Can you work these out from the model? Positions are in its coordinate system, mm. A direction names the side the tool comes from. Give positions to 0.01 mm unless a question says otherwise; leave off trailing zeros. Loops run counter-clockwise (first coordinate to the right, second up) from the corner with the lowest first, then second, coordinate; pieces in that order, holes last.
from build123d import *

# Parameters (mm, degrees)
EXTRUDE_1_DEPTH = 100


with BuildPart() as part:
    # 草图1 → 凸台-拉伸1 (new body)
    with BuildSketch(Plane.XY):
        with BuildLine():
            Line((-4.219496526, 3.940708363), (-77.303320181, 72.195779383))
            ThreePointArc((-77.303320181, 72.195779383), (-80.46030058, 74.190187557), (-84.128827283, 74.887397018))
            Line((-84.128827283, 74.887397018), (-88.128827283, 74.887397018))
            ThreePointArc((-88.128827283, 74.887397018), (-88.835934064, 75.180290236), (-89.128827283, 75.887397018))
            Line((-89.128827283, 75.887397018), (-89.128827283, 78.887397018))
            ThreePointArc((-89.128827283, 78.887397018), (-88.835934064, 79.594503799), (-88.128827283, 79.887397018))
            Line((-88.128827283, 79.887397018), (-84.128827283, 79.887397018))
            ThreePointArc((-84.128827283, 79.887397018), (-78.626037228, 78.841582827), (-73.89056663, 75.849970566))
            Line((-73.89056663, 75.849970566), (-0.806742975, 7.594899545))
            ThreePointArc((-0.806742975, 7.594899545), (1.477574895, 6.378091558), (4.064256195, 6.466463865))
            Line((4.064256195, 6.466463865), (50.410774928, 20.59773729))
            ThreePointArc((50.410774928, 20.59773729), (58.170818827, 20.86285421), (65.023772438, 17.212430248))
            Line((65.023772438, 17.212430248), (82.729423008, 0.676617305))
            Line((82.729423008, 0.676617305), (86.383614191, -2.977573878))
            Line((86.383614191, -2.977573878), (79.316669457, -2.977573878))
            Line((79.316669457, -2.977573878), (61.611018887, 13.558239066))
            ThreePointArc((61.611018887, 13.558239066), (57.042383146, 15.99185504), (51.869020547, 15.815110427))
            Line((51.869020547, 15.815110427), (5.522501814, 1.683837001))
            ThreePointArc((5.522501814, 1.683837001), (0.349139215, 1.507092388), (-4.219496526, 3.940708363))
        make_face()
    extrude(amount=EXTRUDE_1_DEPTH)


solid = part.part
(1) Please list where these lines run through material, in increasing order: probe 1 along Y at (x, z) = (74.5, 71); probe 2 along X at (y, z) = (34.5, 33); probe 3 along Y at (x, z) = (73, 51.5).
Returned:
probe 1: y = 1.52 to 8.36
probe 2: x = -36.94 to -29.62
probe 3: y = 2.92 to 9.76
(2) Suppose I cut it at C-C on y = 57. List the corners of the cut face in (x, z) for me.
Returned:
outline: (-61.03, 0) - (-53.71, 0) - (-53.71, 100) - (-61.03, 100) - close
(3) Suppose I cut it at A-A on z = 15.5. List the corners of the cut face in (x, y) for me.
Returned:
outline: (-89.13, 75.89) arc R1 ccw to (-88.13, 74.89) - (-84.13, 74.89) arc R10 cw to (-77.3, 72.2) - (-4.22, 3.94) arc R10 ccw to (5.52, 1.68) - (51.87, 15.82) arc R10 cw to (61.61, 13.56) - (79.32, -2.98) - (86.38, -2.98) - (82.73, 0.68) - (65.02, 17.21) arc R15 ccw to (50.41, 20.6) - (4.06, 6.47) arc R5 cw to (-0.81, 7.59) - (-73.89, 75.85) arc R15 ccw to (-84.13, 79.89) - (-88.13, 79.89) arc R1 ccw to (-89.13, 78.89) - close
(4) Thinking about a two-plate mould opening in X: for faces 5 (the flat face through (26.913, 13.433, 49.3)), 6 (the flat face through (73.753, 9.06, 49.3)), 7 (the flat face through (-14, 17, 100)), which applies, pulls with the +X half, pulls with the -X half, needs draft (parallel to the pull), parting line crosses it, or undercut?
Returned:
face 5: undercut
face 6: pulls with the +X half
face 7: needs draft
(5) Will these pins go through, and if not, where does the flat tip stop? P1, Ø4, axis at y = 13.5, z = 28, coming from the +X side; P2, Ø10, axis at x = 54.5, z = 90, coming from the -Y side; P3, Ø6, axis at y = 69.5, z = 76, coming from the +X side.
Returned:
P1: stops at x = 71.14
P2: stops at y = 15.07
P3: stops at x = -63.88
(6) Suppose I cut it at B-B on x = 17. List the corners of the cut face in (y, z) for me, plus the area to 3 significant figures.
Returned:
outline: (5.18, 0) - (10.41, 0) - (10.41, 100) - (5.18, 100) - close
area: 523 mm2
(7) Which directions (+Z, -Z, +X, -X, +Y, -Y) give clear straight access to the entire face, cutting with the end or side of a thin tool? Please do faces 1 (the flat face through (-86, 74.887, 49)), 2 (the flat face through (-37.86, 42.2, 49.3)), 3 (the flat face through (-86, 79.887, 49)), 4 (the flat face through (70.59, 5.17, 49.3)).
Returned:
face 1: +Z, -Z, -X, -Y
face 2: +Z, -Z, +Y
face 3: +Z, -Z, +X, -X, +Y
face 4: +Z, -Z, -Y
